Check sheet for the drawn part. Datum: minimum x, y, z corner. Units: mm. A direction names the side the tool comes from. Round coordinates to 2 decimals unless told otherwise and drop trailing zeros. Write each loop counter-clockwise with the first axis right and the second up, starting at its lowest first coordinate (ties: lowest second). Pieces come first, ordered by that corner, then holes. Notation, with made-up numbers: M 5,63 L 39,63 A29 cw 39,95 Z; hole C -34,48 d2. An arc over 180 degrees is marked long. One line per item, written item: value.
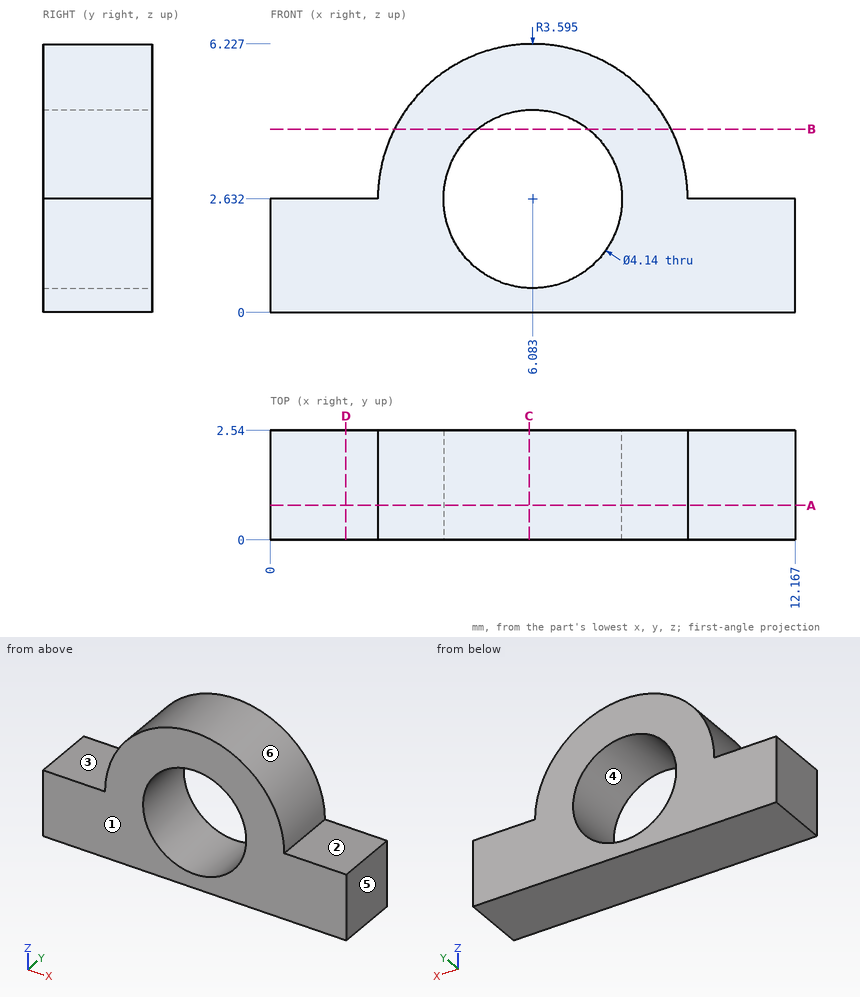
Q1. Sectioned sample at A-A on y = 0.8. Enter the section's corners in (x, z) (1 decimal).
Completed:
outline: M 0,0 L 12.2,0 L 12.2,2.6 L 9.7,2.6 A3.6 ccw 2.5,2.6 L 0,2.6 Z; hole C 6.1,2.6 d4.1
Q2. Sectioned sample at C-C on x = 6. Enter the section's corners in (y, z) (1 decimal).
Completed:
outline: M 0,0 L 2.5,0 L 2.5,0.6 L 0,0.6 Z; M 0,4.7 L 2.5,4.7 L 2.5,6.2 L 0,6.2 Z
Q3. Access from +Z, -Z, +X, -X, +Y, -Y to the whole of each face (thin tool, end or side, straight path). Record for the marked faces 1, 2 and 3.
Completed:
face 1: +Z, -Z, +X, -X, -Y
face 2: +Z, +X, +Y, -Y
face 3: +Z, -X, +Y, -Y
Q4. Draft check along X on the marked faces 4, 5 and 6. Enter one of: pulls with the +X half, pulls with the -X half, needs draft (parallel to the pull), parting line crosses it, or undercut.
Completed:
face 4: undercut
face 5: pulls with the +X half
face 6: parting line crosses it
Q5. Depth check by flat-ended pin: P1, Ø1.2, axis at x = 1.5, y = 1.5, coming from the +Z side. Enter the tip coordinate at first touch or a pass-through.
Completed:
P1: z = 2.63
Q6. Sectioned sample at B-B on z = 4.25. Enter the section's corners in (x, y) (1 decimal).
Completed:
outline: M 2.9,0 L 4.8,0 L 4.8,2.5 L 2.9,2.5 Z; M 7.4,0 L 9.3,0 L 9.3,2.5 L 7.4,2.5 Z
Q7. Sectioned sample at D-D on x = 1.75. Enter the section's corners in (y, z).
Completed:
outline: M 0,0 L 2.54,0 L 2.54,2.63 L 0,2.63 Z
Q8. Scan lines: line 1 (Z direction, x = 6, y = 2.05) (1 decimal); line 2 (Z direction, x = 1, y = 0.95); line 3 (X direction, y = 1.9, z = 3.5) (1 decimal). Record each from-to range of solid material in increasing order. Write a range as [from, to].
Completed:
line 1: [0, 0.6], [4.7, 6.2]
line 2: [0, 2.63]
line 3: [2.6, 4.2], [8, 9.6]
